```python
from build123d import *

# Parameters (mm, degrees)
F0_W     = 48.5
F0_H     = 2.2
F1_DEPTH = 4.5
F2_W     = 1
F2_H     = 1
F3_DEPTH = 4
F4_R     = 0.1
F5_DEPTH = 2.5


with BuildPart() as f1:
    # F0 (on Top) → F1 (new body)
    with BuildSketch(Plane.XY):
        Rectangle(F0_W, F0_H)
    extrude(amount=F1_DEPTH)

    # F2 (on face) → F3 (cut)
    with BuildSketch(Plane.XY.offset(4.5)):
        with Locations((23, 0)):
            Rectangle(F2_W, F2_H)
        with Locations((21, 0)):
            Rectangle(F2_W, F2_H)
        with Locations((19, 0)):
            Rectangle(F2_W, F2_H)
        with Locations((17, 0)):
            Rectangle(F2_W, F2_H)
        with Locations((15, 0)):
            Rectangle(F2_W, F2_H)
        with Locations((13, 0)):
            Rectangle(F2_W, F2_H)
        with Locations((11, 0)):
            Rectangle(F2_W, F2_H)
        with Locations((9, 0)):
            Rectangle(F2_W, F2_H)
        with Locations((7, 0)):
            Rectangle(F2_W, F2_H)
        with Locations((5, 0)):
            Rectangle(F2_W, F2_H)
        with Locations((3, 0)):
            Rectangle(F2_W, F2_H)
        with Locations((1, 0)):
            Rectangle(F2_W, F2_H)
        with Locations((-1, 0)):
            Rectangle(F2_W, F2_H)
        with Locations((-3, 0)):
            Rectangle(F2_W, F2_H)
        with Locations((-5, 0)):
            Rectangle(F2_W, F2_H)
        with Locations((-7, 0)):
            Rectangle(F2_W, F2_H)
        with Locations((-9, 0)):
            Rectangle(F2_W, F2_H)
        with Locations((-11, 0)):
            Rectangle(F2_W, F2_H)
        with Locations((-13, 0)):
            Rectangle(F2_W, F2_H)
        with Locations((-15, 0)):
            Rectangle(F2_W, F2_H)
        with Locations((-17, 0)):
            Rectangle(F2_W, F2_H)
        with Locations((-19, 0)):
            Rectangle(F2_W, F2_H)
        with Locations((-21, 0)):
            Rectangle(F2_W, F2_H)
        with Locations((-23, 0)):
            Rectangle(F2_W, F2_H)
    extrude(amount=-F3_DEPTH, mode=Mode.SUBTRACT)

    # F4 (on face) → F5 (join)
    with BuildSketch(Plane(origin=(0, 0, 0), x_dir=(1, 0, 0), z_dir=(0, 0, -1))):
        with Locations((23, 0)):
            Circle(F4_R)
        with Locations((21, 0)):
            Circle(F4_R)
        with Locations((19, 0)):
            Circle(F4_R)
        with Locations((17, 0)):
            Circle(F4_R)
        with Locations((15, 0)):
            Circle(F4_R)
        with Locations((13, 0)):
            Circle(F4_R)
        with Locations((11, 0)):
            Circle(F4_R)
        with Locations((9, 0)):
            Circle(F4_R)
        with Locations((7, 0)):
            Circle(F4_R)
        with Locations((5, 0)):
            Circle(F4_R)
        with Locations((3, 0)):
            Circle(F4_R)
        with Locations((1, 0)):
            Circle(F4_R)
        with Locations((-1, 0)):
            Circle(F4_R)
        with Locations((-3, 0)):
            Circle(F4_R)
        with Locations((-5, 0)):
            Circle(F4_R)
        with Locations((-7, 0)):
            Circle(F4_R)
        with Locations((-9, 0)):
            Circle(F4_R)
        with Locations((-11, 0)):
            Circle(F4_R)
        with Locations((-13, 0)):
            Circle(F4_R)
        with Locations((-15, 0)):
            Circle(F4_R)
        with Locations((-17, 0)):
            Circle(F4_R)
        with Locations((-19, 0)):
            Circle(F4_R)
        with Locations((-21, 0)):
            Circle(F4_R)
        with Locations((-23, 0)):
            Circle(F4_R)
    extrude(amount=F5_DEPTH)


solid = f1.part
```
Check sheet for the modelled part. Datum: model origin and axes. Units: mm. Round coordinates to 2 decimals unless told otherwise and drop trailing zeros. Order: outer loops, then holes, each group sorted by start corner. A loop starts at its lowest first (then second) coordinate and runs counter-clockwise, first axis right, second up. Notation, with made-up numbers: (-18, -30) -> (1, -30) arc R24 cw to (1, -3) -> close; hole circle Ø2 at (56.25, -31). An arc over 180 degrees is marked (long way). One line per item, written item: value. Start each with the question number.
Q1. Cross-section at B-B (x = -6). Record the boundary of the cut face in (y, z).
Q2. Gauge pin test, flat end, axial feed: pin 1 Ø0.8 at (x, y) = (-9, 0) entering from +Z. Record the tip position at first contact, or that the pin passes through.
Q3. Mould release check, pull along Y, two halves, no side actions. Record for faces 1 (the face through (24.25, 0, 2)), 2 (the face through (8.5, 0, 3)): pulls with the +Y half, pulls with the -Y half, needs draft (parallel to the pull), parting line crosses it, or undercut.
Q4. Thickness scan on line 1 (Y direction, x = -11, z = 1); line 2 (Z direction, x = 15.5, y = -0.7); line 3 (Z direction, x = 19, y = 0.4). Record the ranges inside material, lowest first.
Q5. Cross-section at A-A (z = -0.75). Give the number of separate pieces and of enclosed holes in the cut face, and give its area (3 significant figures).
Completed:
1. outline: (-1.1, 0) -> (1.1, 0) -> (1.1, 4.5) -> (-1.1, 4.5) -> close
2. pin 1: stops at z = 0.5
3. face 1: needs draft
3. face 2: undercut
4. line 1: y = -1.1 to -0.5, 0.5 to 1.1
4. line 2: z = 0 to 4.5
4. line 3: z = 0 to 0.5
5. separate pieces: 24
5. enclosed holes: 0
5. area: 0.754 mm²
